from build123d import *

# Parameters (mm, degrees)
SKETCH2_W          = 31.114715918
SKETCH2_H          = 104.73171331
CUT_EXTRUDE1_DEPTH = 48


with BuildPart() as part:
    # Sketch1 → Revolve1 (revolve)
    with BuildSketch(Plane.YZ, mode=Mode.PRIVATE) as revolve1_sk:
        with BuildLine():
            Line((0, 0), (17.5, 0))
            ThreePointArc((17.5, 0), (28.106601718, 4.393398282), (32.5, 15))
            Line((32.5, 15), (32.5, 140.55339898))
            ThreePointArc((32.5, 140.55339898), (31.881408374, 144.816624656), (30.076654245, 148.728224239))
            Line((30.076654245, 148.728224239), (18.673345755, 166.271775761))
            ThreePointArc((18.673345755, 166.271775761), (16.868591626, 170.183375344), (16.25, 174.44660102))
            Line((16.25, 174.44660102), (16.25, 190))
            Line((16.25, 190), (0, 190))
            Line((0, 190), (0, 189))
            Line((0, 189), (15.25, 189))
            Line((15.25, 189), (15.25, 174.44660102))
            ThreePointArc((15.25, 174.44660102), (15.909831067, 169.899160298), (17.834902139, 165.72678741))
            Line((17.834902139, 165.72678741), (29.238210628, 148.183235889))
            ThreePointArc((29.238210628, 148.183235889), (30.922647816, 144.532409611), (31.5, 140.55339898))
            Line((31.5, 140.55339898), (31.5, 15))
            ThreePointArc((31.5, 15), (27.399494937, 5.100505063), (17.5, 1))
            Line((17.5, 1), (0, 1))
            Line((0, 1), (0, 0))
        make_face()
    revolve(revolve1_sk.sketch.rotate(Axis((0, 0, 0), (0, 0, 1)), 90), axis=Axis((0, 0, 0), (0, 0, 1)))

    # Sketch2 → Cut-Extrude1 (cut)
    with BuildSketch(Plane.YZ.offset(60)):
        with Locations((0.396690762, 79.674592023)):
            Rectangle(SKETCH2_W, SKETCH2_H)
    extrude(amount=-CUT_EXTRUDE1_DEPTH, mode=Mode.SUBTRACT)


solid = part.part
Read the model definition and answer for the solid it produces. Units are mm, in the model's axes. A direction names the side the tool comes from. Give positions to 0.01 mm unless a question says otherwise; leave off trailing zeros. Loops run counter-clockwise (first coordinate to the right, second up) from the corner with the lowest first, then second, coordinate; pieces in that order, holes last. Notation, with made-up numbers: (33, 75) -> (79, 75) arc R22 ccw to (79, 95) -> close; hole circle Ø10 at (72, -13). An arc over 180 degrees is marked (long way). Answer as CSV lines item,"result".
Item 1: For faces 4 (the face through (-31, -9.76, 78.66)), 5 (the face through (-30.045, -9.462, 76.898)), 6 (the face through (-15.5, -4.88, 182.33)), determine the directions among +Z, -Z, +X, -X, +Y, -Y from which every point of the face is accessible in a straight line to the end or side of a thin tool.
Returned:
face 4,"+Z, -Z"
face 5,"none"
face 6,"+Z"
Item 2: Each of these flat-tipped pins is pushed along its axis until it touches: pin 1 (1 mm diameter, centred on x = -3.5, y = -25, fed in from +Z); pin 2 (2.5 mm diameter, centred on x = 29.5, y = 7, fed in from -Z); pin 3 (0.6 mm diameter, centred on x = 28, z = 63.5, fed in from +Y). Where does it stop, or does it pass through?
Returned:
pin 1,"stops at z = 156.93"
pin 2,"stops at z = 5.45"
pin 3,"stops at y = 17"
Item 3: Find section A-A on x = 0. Give the vertices of the cut face in (y, z).
Returned:
outline,"(-32.5, 15) arc R15 ccw to (-17.5, 0) -> (17.5, 0) arc R15 ccw to (32.5, 15) -> (32.5, 140.55) arc R15 ccw to (30.08, 148.73) -> (18.67, 166.27) arc R15 cw to (16.25, 174.45) -> (16.25, 190) -> (-16.25, 190) -> (-16.25, 174.45) arc R15 cw to (-18.67, 166.27) -> (-30.08, 148.73) arc R15 ccw to (-32.5, 140.55) -> close; hole (-31.5, 15) arc R14 ccw to (-17.5, 1) -> (17.5, 1) arc R14 ccw to (31.5, 15) -> (31.5, 140.55) arc R14 ccw to (29.24, 148.18) -> (17.83, 165.73) arc R16 cw to (15.25, 174.45) -> (15.25, 189) -> (-15.25, 189) -> (-15.25, 174.45) arc R16 cw to (-17.83, 165.73) -> (-29.24, 148.18) arc R14 ccw to (-31.5, 140.55) -> close"
Item 4: Determine the mould class of faces 1 (the face through (0, 0, 190)), 2 (the face through (0, 0, 0)), 3 (the face through (32, 0, 132.04)) for opening direction Z: +Z half, -Z half, draft (parallel to the pull), parting line (faces both ways), or undercut.
Returned:
face 1,"+Z half"
face 2,"-Z half"
face 3,"undercut"
Item 5: Find section D-D on z = 78.5. Give the vertices of the cut face in (x, y), plus the area to 3 significant figures.
Returned:
outline,"(27.16, 15.95) -> (28.31, 15.95) arc R32.5 ccw (long way) to (28.75, -15.16) -> (27.61, -15.16) arc R31.5 cw (long way) to start"
area,"169 mm²"
Item 6: Find section C-C on z = 136. Give the vertices of the cut face in (x, y).
Returned:
outline,"circle Ø65 at (0, 0); hole circle Ø63 at (0, 0)"
Item 7: Consider line 1 (Z direction, x = 14.5, y = 3.5); line 2 (Y direction, x = 0, z = 185.5); line 3 (Z direction, x = 17, y = -7). Determine where each line is inside the solid, lowest interval first. Write a range as [from, to].
Returned:
line 1,"z = [0, 1], [189, 190]"
line 2,"y = [-16.25, -15.25], [15.25, 16.25]"
line 3,"z = [0.03, 1.03], [164.88, 166.73]"
